Read the model definition and answer for the solid it produces. Units are mm, in the model's axes. A direction names the side the tool comes from. Coordinates: 2 decimals unless noted, no trailing zeros. Loops run counter-clockwise (first coordinate to the right, second up) from the corner with the lowest first, then second, coordinate; pieces in that order, holes last. Notation, with made-up numbers: M -30,85 L -3,85 A21 cw -3,92 Z; hole C 6,-6 d11. An arc over 180 degrees is marked long. One line per item, written item: value. Start each with the question number.
1. The part is cut by section A-A (y = -4.5). Write down the section's boundary in (x, z).
2. Consider probe 1 along Y at (x, z) = (-60.25, 0); probe 2 along X at (y, z) = (0.75, 6.25); probe 3 along Z at (x, y) = (42, -0.5). Determine where each line is inside the solid, lowest interval first.
3. For faces 1 (the face through (-69.799, 0, -3)), 2 (the face through (70.52, 5.669, 1.785)), determine the directions among +Z, -Z, +X, -X, +Y, -Y from which every point of the face is accessible in a straight line to the end or side of a thin tool.
4. The part is cut by section B-B (x = 60). Write down the section's boundary in (y, z).
5. Determine the mould class of faces 3 (the face through (-52.02, -0.17, 0.41)), 4 (the face through (80.61, -6.2, 1.38)), 5 (the face through (90.272, 0, 0)), 6 (the face through (-61.429, 0.767, -2.435)) for opening direction Y: +Y half, -Y half, draft (parallel to the pull), parting line (faces both ways), or undercut.
6. Flat-ended cylindrical pins translate along their axes: pin 1 (3 mm diameter, centred on x = -29.5, z = 3.5, fed in from -Y); pin 2 (2 mm diameter, centred on x = 48.5, y = -5, fed in from -Z). Find the tip coordinate at first contact, or state that the pin passes through.
```python
from build123d import *

# Parameters (mm, degrees)
SKETCH1_R                   = 6.35
BOSS_EXTRUDE1_DEPTH         = 69.7992
SKETCH2_W                   = 1.4224
SKETCH2_H                   = 5.9436
SKETCH3_R                   = 6.35
BOSS_EXTRUDE2_DEPTH         = 19.05
F_1_4_20_TAPPED_HOLE1_D     = 5.1054
F_1_4_20_TAPPED_HOLE1_DEPTH = 16.51
F_1_4_20_TAPPED_HOLE1_TIP   = 1.533816902


with BuildPart() as part:
    # Sketch1 → Boss-Extrude1 (new body, symmetric)
    with BuildSketch(Plane(origin=(0, 0, 0), x_dir=(0, 0, -1), z_dir=(1, 0, 0))):
        Circle(SKETCH1_R)
    extrude(amount=BOSS_EXTRUDE1_DEPTH, both=True)

    # Sketch2 → Revolve2 (revolve)
    with BuildSketch(Plane.XY):
        with Locations((70.5104, 2.9718)):
            Rectangle(SKETCH2_W, SKETCH2_H)
    revolve(axis=Axis((0, 0, 0), (1, 0, 0)))

    # Sketch3 → Boss-Extrude2 (add)
    with BuildSketch(Plane(origin=(71.2216, 0, 0), x_dir=(0, 0, -1), z_dir=(1, 0, 0))):
        Circle(SKETCH3_R)
    extrude(amount=BOSS_EXTRUDE2_DEPTH)

    # 1/4-20 Tapped Hole1
    with Locations(Plane.ZY.offset(69.7992)):
        with Locations((0, 0)):
            Hole(F_1_4_20_TAPPED_HOLE1_D / 2, depth=F_1_4_20_TAPPED_HOLE1_DEPTH)
            with Locations((0, 0, -(F_1_4_20_TAPPED_HOLE1_DEPTH + F_1_4_20_TAPPED_HOLE1_TIP / 2))):  # 118° drill point
                Cone(0, F_1_4_20_TAPPED_HOLE1_D / 2, F_1_4_20_TAPPED_HOLE1_TIP, mode=Mode.SUBTRACT)


solid = part.part
```
Answer block:
1. outline: M -69.8,-4.48 L 69.8,-4.48 L 69.8,-3.88 L 71.22,-3.88 L 71.22,-4.48 L 90.27,-4.48 L 90.27,4.48 L 71.22,4.48 L 71.22,3.88 L 69.8,3.88 L 69.8,4.48 L -69.8,4.48 Z
2. probe 1: y = -6.35 to -2.55, 2.55 to 6.35
2. probe 2: x = -69.8 to 69.8, 71.22 to 90.27
2. probe 3: z = -6.33 to 6.33
3. face 1: +Z, -Z, -X, +Y, -Y
3. face 2: none
4. outline: C 0,0 d12.7
5. face 3: undercut
5. face 4: parting line
5. face 5: draft
5. face 6: undercut
6. pin 1: stops at y = -6.03
6. pin 2: stops at z = -4.93
